from build123d import *

# Parameters (mm, degrees)
BOSS_EXTRUDE1_DEPTH      = 20
CUT_EXTRUDE1_DEPTH       = 2
M3_CLEARANCE_HOLE1_D     = 3.6
M3_CLEARANCE_HOLE1_DEPTH = 3


with BuildPart() as part:
    # Sketch1 → Boss-Extrude1 (new body)
    with BuildSketch(Plane.XY):
        with BuildLine():
            Line((-22.5, 19), (-11.2, 19))
            Line((-11.2, 19), (-11.2, 16.8))
            Line((-11.2, 16.8), (-14.700438244, 14.2))
            Line((-14.700438244, 14.2), (-14.396845337, -0.301403929))
            ThreePointArc((-14.396845337, -0.301403929), (0, -14.4), (14.396845337, -0.301403929))
            Line((14.396845337, -0.301403929), (14.700438244, 14.2))
            Line((14.700438244, 14.2), (11.2, 16.8))
            Line((11.2, 16.8), (11.2, 19))
            Line((11.2, 19), (22.5, 19))
            Line((22.5, 19), (22.5, 22))
            Line((22.5, 22), (9.2, 22))
            Line((9.2, 22), (9.2, 16.799674488))
            Line((9.2, 16.799674488), (12.7, 14.2))
            Line((12.7, 14.2), (12.397283485, -0.259542272))
            ThreePointArc((12.397283485, -0.259542272), (0, -12.4), (-12.397283485, -0.259542272))
            Line((-12.397283485, -0.259542272), (-12.7, 14.2))
            Line((-12.7, 14.2), (-9.2, 16.799674488))
            Line((-9.2, 16.799674488), (-9.2, 22))
            Line((-9.2, 22), (-22.5, 22))
            Line((-22.5, 22), (-22.5, 19))
        make_face()
    extrude(amount=BOSS_EXTRUDE1_DEPTH)

    # Sketch4 → Cut-Extrude1 (cut)
    with BuildSketch(Plane.XZ.offset(-19)):
        Polygon((-13.41228676, 2.25), (-11.824573519, 5), (-13.41228676, 7.75), (-16.58771324, 7.75), (-18.175426481, 5), (-16.58771324, 2.25), align=None)
        Polygon((-11.824573519, 15), (-13.41228676, 17.75), (-16.58771324, 17.75), (-18.175426481, 15), (-16.58771324, 12.25), (-13.41228676, 12.25), align=None)
        Polygon((13.41228676, 12.25), (11.824573519, 15), (13.41228676, 17.75), (16.58771324, 17.75), (18.175426481, 15), (16.58771324, 12.25), align=None)
        Polygon((16.58771324, 2.25), (13.41228676, 2.25), (11.824573519, 5), (13.41228676, 7.75), (16.58771324, 7.75), (18.175426481, 5), align=None)
    extrude(amount=-CUT_EXTRUDE1_DEPTH, mode=Mode.SUBTRACT)

    # M3 Clearance Hole1
    with Locations(Plane(origin=(0, 19, 0), x_dir=(-1, 0, 0), z_dir=(0, -1, 0))):
        with Locations((-15, -15), (15, -15), (-15, -5), (15, -5)):
            Hole(M3_CLEARANCE_HOLE1_D / 2, depth=M3_CLEARANCE_HOLE1_DEPTH)


solid = part.part
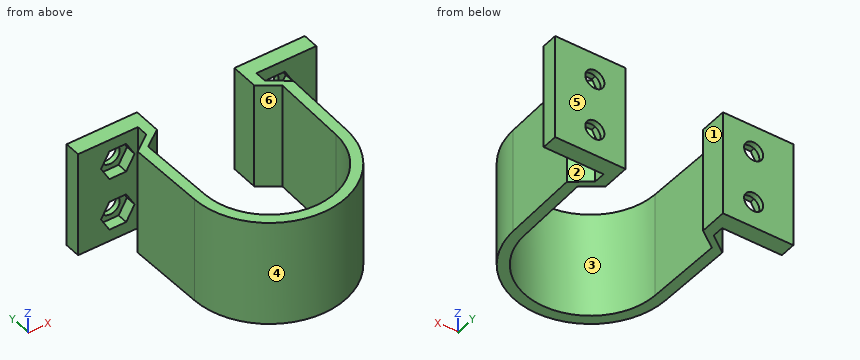
Source: CAD feature listing. Evaluate the final solid. Frame: model axes, mm. Face numbers are marked on the shaded views. A direction names the side the tool comes from. Round coordinates to 2 decimals unless told otherwise and drop trailing zeros. Write each loop counter-clockwise with the first axis right and the second up, starting at its lowest first coordinate (ties: lowest second). Pieces come first, ordered by that corner, then holes. Notation, with made-up numbers: M 22.25,3 L 56.25,3 A24 cw 56.25,13 Z; hole C 58,12.5 d4. An arc over 180 degrees is marked long. One line per item, written item: value. Start each with the question number.
Item 1: Section query D-D (x = -19). Return the cut outline in (y, z).
Item 2: Section query B-B (x = 10). Return the cut outline in (y, z), plus the area to 3 significant figures.
Item 3: Section query C-C (z = 18.5). Return the cut outline in (x, y).
Item 4: Section query A-A (y = -6.5). Return the cut outline in (x, z).
Item 5: Pin query (flat end, axial travel): pin 1 (3 mm diameter, centred on x = 14, z = 14, fed in from -Y); pin 2 (1.5 mm diameter, centred on y = 3, z = 6, fed in from -X); pin 3 (9 mm diameter, centred on x = 17.5, z = 11, fed in from -Y). Return the tip coordinate at first contact, or that it passes through.
Item 6: Set-up query: the marked faces 1, 2 and 3. Return all of +Z, -Z, +X, -X, +Y, -Y with unobstructed straight access to the full face (end or side cutting, diameter ignored); none if empty.
Item 7: Ray query, L1, parallel to X at y = 21.35, z = 5; L2, parallel to Z at x = -15, y = 21.65; L3, parallel to X at y = 0, z = 1. Return the intervals inside material, ascending. Write a range as from..to.
Item 8: Mould query, pull axis X, two halves, no side actions, for the marked faces 4, 5 and 6. Classes: pulls with the +X half, pulls with the -X half, needs draft (parallel to the pull), parting line crosses it, or undercut.
Result set:
1. outline: M 19,0 L 22,0 L 22,20 L 19,20 Z
2. outline: M -10.36,0 L -7.33,0 L -7.33,20 L -10.36,20 Z; M 16.21,0 L 22,0 L 22,20 L 16.21,20 Z
2. area: 176 mm²
3. outline: M -22.5,19 L -11.2,19 L -11.2,16.8 L -14.7,14.2 L -14.4,-0.3 A14.4 ccw 14.4,-0.3 L 14.7,14.2 L 11.2,16.8 L 11.2,19 L 22.5,19 L 22.5,22 L 9.2,22 L 9.2,16.8 L 12.7,14.2 L 12.4,-0.26 A12.4 cw -12.4,-0.26 L -12.7,14.2 L -9.2,16.8 L -9.2,22 L -22.5,22 Z
4. outline: M -12.85,0 L -10.56,0 L -10.56,20 L -12.85,20 Z; M 10.56,0 L 12.85,0 L 12.85,20 L 10.56,20 Z
5. pin 1: stops at y = -7.15
5. pin 2: stops at x = -14.48
5. pin 3: stops at y = -6.19
6. face 1: +Z, -Z, +Y
6. face 2: +Z, -Z, +X
6. face 3: +Z, -Z
7. L1: x = -22.5..-16.8, -13.2..-9.2, 9.2..13.2, 16.8..22.5
7. L2: z = 0..3.2, 6.8..13.2, 16.8..20
7. L3: x = -14.4..-12.4, 12.4..14.4
8. face 4: parting line crosses it
8. face 5: needs draft
8. face 6: undercut
